Design review of the part built by this model. Coordinates are the model's own, in mm. Face numbers are marked on the shaded views. A direction names the side the tool comes from. Round coordinates to 2 decimals unless told otherwise and drop trailing zeros. Order: outer loops, then holes, each group sorted by start corner. A loop starts at its lowest first (then second) coordinate and runs counter-clockwise, first axis right, second up. Notation, with made-up numbers: (29.5, -29.75) - (44.5, -29.75) arc R20 ccw to (44.5, 6.25) - close; hole circle Ø2 at (-17.5, -27). An arc over 180 degrees is marked (long way). Write item = value, one per line.
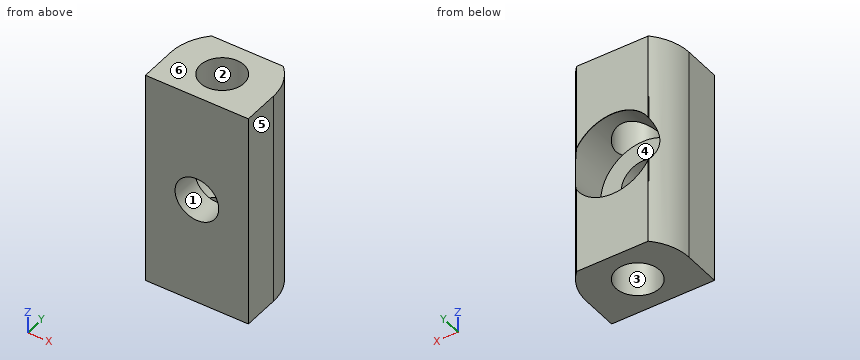
from build123d import *

# Parameters (mm, degrees)
SKETCH2_R             = 3.475
BOSS_EXTRUDE2_DEPTH   = 14.575
SKETCH3_R             = 1.475
CUT_EXTRUDE1_DEPTH    = 10
CUT_EXTRUDE2_START    = -10
SKETCH4_R             = 1.475
CUT_EXTRUDE2_DEPTH    = 10
BOSS_EXTRUDE3_DEPTH   = 14.575
SKETCH6_W             = 6.95
SKETCH6_H             = 14.575
BOSS_EXTRUDE4_DEPTH   = 0.2
SKETCH8_W             = 6
SKETCH8_H             = 2
CUT_EXTRUDE3_DEPTH    = 17.560155
SKETCH10_R            = 2.85
CUT_EXTRUDE4_DEPTH    = 3
SKETCH11_R            = 1.675
CUT_EXTRUDE5_DEPTH    = 16.508264
SKETCH17_R            = 2.85
BOSS_EXTRUDE8_DEPTH   = 3.15
BOSS_EXTRUDE9_DEPTH   = 0.150002
BOSS_EXTRUDE9_START   = 4.437502
BOSS_EXTRUDE9_2_DEPTH = 1.376058
BOSS_EXTRUDE9_START_2 = 2.475
BOSS_EXTRUDE9_3_DEPTH = 1.525
BOSS_EXTRUDE12_START  = 4
BOSS_EXTRUDE12_DEPTH  = 4
CUT_EXTRUDE6_DEPTH    = 17.322741
SKETCH23_R            = 1.475
CUT_EXTRUDE8_DEPTH    = 16.508264
SKETCH24_W            = 6.95
SKETCH24_H            = 1.175
CUT_EXTRUDE9_DEPTH    = 16.427634


with BuildPart() as part:
    # Sketch2 → Boss-Extrude2 (new body)
    with BuildSketch(Plane.XY):
        Circle(SKETCH2_R)
    extrude(amount=BOSS_EXTRUDE2_DEPTH)

    # Sketch3 → Cut-Extrude1 (cut)
    with BuildSketch(Plane.XY.offset(14.575)):
        Circle(SKETCH3_R)
    extrude(amount=-CUT_EXTRUDE1_DEPTH, mode=Mode.SUBTRACT)

    # Sketch4 → Cut-Extrude2 (cut)
    with BuildSketch(Plane(origin=(0, 0, 0), x_dir=(-1, 0, 0), z_dir=(0, 0, -1)).offset(CUT_EXTRUDE2_START)):
        with Locations(Location((0, 0, 0), (0, 0, 180))):
            Circle(SKETCH4_R)
    extrude(amount=CUT_EXTRUDE2_DEPTH, mode=Mode.SUBTRACT)

    # Sketch5 → Boss-Extrude3 (add)
    with BuildSketch(Plane(origin=(0, 0, 0), x_dir=(-1, 0, 0), z_dir=(0, 0, -1))):
        with BuildLine():
            ThreePointArc((0, -3.475), (-2.457196, -2.457196), (-3.475, 0))
            Line((-3.475, 0), (-3.475, -3.475))
            Line((-3.475, -3.475), (0, -3.475))
        make_face()
        with BuildLine():
            Line((3.475, -3.475), (3.475, 0))
            ThreePointArc((3.475, 0), (2.457196, -2.457196), (0, -3.475))
            Line((0, -3.475), (3.475, -3.475))
        make_face()
    extrude(amount=-BOSS_EXTRUDE3_DEPTH)

    # Sketch6 → Boss-Extrude4 (add)
    with BuildSketch(Plane.XZ.offset(3.475)):
        with Locations((0, 7.2875)):
            Rectangle(SKETCH6_W, SKETCH6_H)
    extrude(amount=BOSS_EXTRUDE4_DEPTH)

    # Sketch8 → Cut-Extrude3 (cut, through all)
    with BuildSketch(Plane.ZY.offset(3.475)):
        with Locations((7.2875, 3.475)):
            Rectangle(SKETCH8_W, SKETCH8_H)
    extrude(amount=-CUT_EXTRUDE3_DEPTH, mode=Mode.SUBTRACT)

    # Sketch10 → Cut-Extrude4 (cut)
    with BuildSketch(Plane(origin=(0, 2.475, 0), x_dir=(1, 0, 0), z_dir=(0, 1, 0))):
        with Locations(Location((0, -7.2875, 0), (0, 0, 298.924116))):
            Circle(SKETCH10_R)
    extrude(amount=-CUT_EXTRUDE4_DEPTH, mode=Mode.SUBTRACT)

    # Sketch11 → Cut-Extrude5 (cut, through all)
    with BuildSketch(Plane(origin=(0, -0.525, 0), x_dir=(1, 0, 0), z_dir=(0, 1, 0))):
        with Locations(Location((0, -7.2875, 0), (0, 0, 270))):
            Circle(SKETCH11_R)
    extrude(amount=-CUT_EXTRUDE5_DEPTH, mode=Mode.SUBTRACT)

    # Sketch17 → Boss-Extrude8 (add)
    with BuildSketch(Plane(origin=(0, -0.525, 0), x_dir=(1, 0, 0), z_dir=(0, 1, 0))):
        with Locations(Location((0, -7.2875, 0), (0, 0, 298.924116))):
            Circle(SKETCH17_R)
    extrude(amount=-BOSS_EXTRUDE8_DEPTH)

    # Boss-Extrude9: read off the stored shape, not the designer's step
    # Boss-Extrude9 outline → Boss-Extrude9 (add)
    with BuildSketch(Plane.XY.offset(4.2875)):
        with BuildLine():
            ThreePointArc((2.439262, 2.475), (0, 3.475), (-2.439262, 2.475))
            Line((-2.439262, 2.475), (2.439262, 2.475))
        make_face()
    extrude(amount=BOSS_EXTRUDE9_DEPTH)

    # Boss-Extrude9 2 outline → Boss-Extrude9 2 (add)
    with BuildSketch(Plane.XY.offset(BOSS_EXTRUDE9_START)):
        with BuildLine():
            ThreePointArc((2.439262, 2.475), (0, 3.475), (-2.439262, 2.475))
            Line((-2.439262, 2.475), (2.439262, 2.475))
        make_face()
    extrude(amount=BOSS_EXTRUDE9_2_DEPTH)

    # Boss-Extrude9 3 outline → Boss-Extrude9 3 (cut)
    with BuildSketch(Plane(origin=(0, 0, 0), x_dir=(1, 0, 0), z_dir=(0, 1, 0)).offset(BOSS_EXTRUDE9_START_2)):
        with BuildLine():
            ThreePointArc((-0.003518, -4.437502), (-1.401848, -4.806105), (-2.439262, -5.81356))
            Line((-2.439262, -5.81356), (2.439262, -5.81356))
            ThreePointArc((2.439262, -5.81356), (1.401848, -4.806105), (0.003518, -4.437502))
            Line((0.003518, -4.437502), (-0.003518, -4.437502))
        make_face()
    extrude(amount=BOSS_EXTRUDE9_3_DEPTH, mode=Mode.SUBTRACT)

    # Sketch20 → Boss-Extrude12 (add)
    with BuildSketch(Plane(origin=(0, 2.475, 0), x_dir=(1, 0, 0), z_dir=(0, 1, 0)).offset(BOSS_EXTRUDE12_START)):
        with BuildLine():
            Line((-2.439262, -10.2875), (2.439262, -10.2875))
            Line((2.439262, -10.2875), (2.439262, -8.76144))
            ThreePointArc((2.439262, -8.76144), (0, -10.1375), (-2.439262, -8.76144))
            Line((-2.439262, -8.76144), (-2.439262, -10.2875))
        make_face()
    extrude(amount=-BOSS_EXTRUDE12_DEPTH)

    # Sketch21 → Cut-Extrude6 (cut, through all)
    with BuildSketch(Plane.XY.offset(14.575)):
        with BuildLine():
            Line((-2.995994, 6.810074), (-2.799337, 2.058965))
            ThreePointArc((-2.799337, 2.058965), (-0.143714, 3.472027), (2.619604, 2.283265))
            Line((2.619604, 2.283265), (3.825654, 6.913781))
            Line((3.825654, 6.913781), (-2.995994, 6.810074))
        make_face()
    extrude(amount=-CUT_EXTRUDE6_DEPTH, mode=Mode.SUBTRACT)

    # Sketch23 → Cut-Extrude8 (cut, through all)
    with BuildSketch(Plane(origin=(0, -0.525, 0), x_dir=(1, 0, 0), z_dir=(0, 1, 0))):
        with Locations(Location((0, -7.2875, 0), (0, 0, 270))):
            Circle(SKETCH23_R)
    extrude(amount=-CUT_EXTRUDE8_DEPTH, mode=Mode.SUBTRACT)

    # Sketch24 → Cut-Extrude9 (cut, through all)
    with BuildSketch(Plane.XY.offset(14.575)):
        with BuildLine():
            ThreePointArc((2.413633, 2.5), (0, 3.475), (-2.413633, 2.5))
            Line((-2.413633, 2.5), (2.413633, 2.5))
        make_face()
        with Locations((0, -3.0875)):
            Rectangle(SKETCH24_W, SKETCH24_H)
    extrude(amount=-CUT_EXTRUDE9_DEPTH, mode=Mode.SUBTRACT)


solid = part.part
Item 1: Insertion check: P1, Ø2.5, axis at x = 0, y = 0, coming from the -Z side. The pin has a flat end and moves straight along its axis. Give the tip position at first contact, or say it passes through.
Data:
P1 = 4.44
Item 2: Take a section at B-B, the plane x = 0.5. State the section outline as (y, z) points (3 decimals).
Data:
outline = (-2.5, 0) - (-1.388, 0) - (-1.388, 4.482) - (-0.525, 4.482) - (-0.525, 5.9) - (-2.5, 5.9) - close; (-2.5, 8.675) - (-0.525, 8.675) - (-0.525, 10.093) - (-1.388, 10.093) - (-1.388, 14.575) - (-2.5, 14.575) - close; (1.388, 0) - (2.5, 0) - (2.5, 4.482) - (1.388, 4.482) - close; (1.388, 10.093) - (2.5, 10.093) - (2.5, 14.575) - (1.388, 14.575) - close
Item 3: The part is to be moulded in two halves that separate along Z. For the marked faces 4, 5 and 6, say which applies: +Z half, -Z half, draft (parallel to the pull), parting line (faces both ways), or undercut.
Data:
face_4 = undercut
face_5 = draft
face_6 = +Z half
Item 4: For line 1 along Y through (x, z) = (0, 11.15) (3 decimals); line 2 along X through (y, z) = (0.1, 2.5); line 3 along Z through (x, y) = (0, 1.85) (1 decimal), list the stretches that pass through material, from the lowest coordinate up. Write a range as [from, to].
Data:
line_1 = [-2.5, -1.475], [1.475, 2.5]
line_2 = [-3.47, -1.47], [1.47, 3.47]
line_3 = [0, 4.4], [10.1, 14.6]
Item 5: Take a section at A-A, the plane z = 3.5. State the section outline as (x, y) points (3 decimals), and give its area (3 significant figures).
Data:
outline = (-3.475, -2.5) - (3.475, -2.5) - (3.475, 0) arc R3.475 ccw to (2.414, 2.5) - (-2.414, 2.5) arc R3.475 ccw to (-3.475, 0) - close; hole circle Ø2.95 at (0, 0)
area = 26.3 mm2
Item 6: For the marked faces 1, 2 and 3, list the 3-axis set-ups (+Z, -Z, +X, -X, +Y, -Y) from which the entire face can be reached by the end or side of a thin tool; tool diameter is ignored.
Data:
face_1 = +Y, -Y
face_2 = +Z
face_3 = -Z
